Work out the finished part from the listing and answer in its coordinate system (mm). Round coordinates to 2 decimals unless told otherwise and drop trailing zeros. Write each loop counter-clockwise with the first axis right and the second up, starting at its lowest first coordinate (ties: lowest second). Pieces come first, ordered by that corner, then holes.
1. Find section B-B (y = -2). Write down the section's boundary in (x, z), and give its area (3 significant figures).
2. Find section C-C (z = 1.75). Count the separate pieces of the cut face and the enclosed holes in it, and give its area (3 significant figures).
3. Find section A-A (x = -27.5). Write down the section's boundary in (y, z).
4. Determine the mould class of faces 1 (the face through (-1, 23, 3)), 2 (the face through (-26.577, 29.726, 1.521)) for opening direction X: pulls with the +X half, pulls with the -X half, needs draft (parallel to the pull), parting line crosses it, or undercut.
5. Straight lines are drawn through the part: probe 1 along Y at (x, z) = (12, 1.15); probe 2 along X at (y, z) = (13, 2.75); probe 3 along Y at (x, z) = (-90, 1.2). For each, find the intervals that lie inside material, in ascending order.
Autodesk Inventor part; units mm, degrees
ref_plane "YZ Plane" through (0, 0, 0) normal (1, 0, 0) x (0, 1, 0)
ref_plane "XZ Plane" through (0, 0, 0) normal (0, 1, 0) x (-1, 0, 0)
ref_plane "XY Plane" through (0, 0, 0) normal (0, 0, 1) x (1, 0, 0)
sketch "Эскиз1" plane through (0, 0, 0) normal (0, 0, 1) x (1, 0, 0)
  line L0 (-100, -50) -> (100, -50)
  line L1 (100, -50) -> (100, 50)
  line L2 (100, 50) -> (-100, 50)
  line L3 (-100, 50) -> (-100, -50)
  line L4 (-100, -50) -> (100, 50) construction
  line L5 (100, -50) -> (-100, 50) construction
  line L6 (-45, -15) -> (45, -15) construction
  line L7 (45, -15) -> (45, 15) construction
  line L8 (45, 15) -> (-45, 15) construction
  line L9 (-45, 15) -> (-45, -15) construction
  line L10 (-45, -15) -> (45, 15) construction
  line L11 (45, -15) -> (-45, 15) construction
  line L12 (0, 15) -> (0, 18) construction
  line L13 (-45, 15) -> (-48, 15) construction
  line L14 (48, -18) -> (-48, -18)
  line L15 (-48, -18) -> (-48, 18)
  line L16 (-48, 18) -> (48, 18)
  line L17 (48, 18) -> (48, -18)
  line L18 (48, -18) -> (-48, 18) construction
  line L19 (-48, -18) -> (48, 18) construction
  point P0 (0, 0)
  dimension "d0" = 200
  dimension "d1" = 100
  dimension "d2" = 90
  dimension "d3" = 30
  dimension "d4" = 3
  dimension "d5" = 3
extrude "Выдавливание1" add sketch "Эскиз1" along normal blind 3
ref_plane "РабПлоскость1" through (0, -50, 0) normal (1, 0, 0) x (0, 0, -1)
sketch "Эскиз2" plane through (0, 0, 3) normal (0, 0, 1) x (1, 0, 0)
  line L0 (-48, -18) -> (-48, 18)
  line L1 (-48, 18) -> (48, 18)
  line L2 (48, 18) -> (48, -18)
  line L3 (48, -18) -> (-48, -18)
  line L4 (-100, -50) -> (100, -50)
  line L5 (100, -50) -> (100, 50)
  line L6 (100, 50) -> (-100, 50)
  line L7 (-100, 50) -> (-100, -50)
  line L8 (48, 18) -> (33.5, 18) construction
  line L9 (33.5, 18) -> (33.5, 50) construction
  line L10 (33.5, 18) -> (27.5, 18) construction
  line L11 (48, 18) -> (-48, 18) construction
  line L12 (27.5, 18) -> (27.5, 50) construction
  line L13 (100, 50) -> (-100, 50) construction
  line L14 (27.5, 18) -> (27.5, 24) construction
  circle A0 centre (27.5, 24) radius 2
  circle A1 centre (27.5, 31.5) radius 2
  circle A2 centre (27.5, 39) radius 2
  line L15 (0, 18) -> (0, 50)
  line L16 (-33.5, 18) -> (-27.5, 18) construction
  line L17 (-27.5, 18) -> (-27.5, 24) construction
  circle A3 centre (-27.5, 24) radius 2
  circle A4 centre (-27.5, 31.5) radius 2
  circle A5 centre (-27.5, 39) radius 2
  point P0 (0, 0)
  dimension "d8" = 14.5
  dimension "d9" = 6
  dimension "d10" = 6
  dimension "d11" = 4
  dimension "d14" = 7.5
extrude "Выдавливание2" cut sketch "Эскиз2" against normal blind 10 contours A0 | A1 | A2 | A3 | A4 | A5
sketch "Эскиз3" plane through (0, 0, 3) normal (0, 0, 1) x (1, 0, 0)
  circle A0 centre (-27.5, 31.5) radius 2
  circle A1 centre (27.5, 39) radius 2
  circle A2 centre (27.5, 24) radius 2
  circle A3 centre (27.5, 31.5) radius 2
  circle A4 centre (-27.5, 24) radius 2
  circle A5 centre (-27.5, 39) radius 2
  line L0 (-48, -18) -> (-48, 18)
  line L1 (-48, 18) -> (48, 18)
  line L2 (48, 18) -> (48, -18)
  line L3 (48, -18) -> (-48, -18)
  line L4 (-100, -50) -> (100, -50)
  line L5 (100, -50) -> (100, 50)
  line L6 (100, 50) -> (-100, 50)
  line L7 (-100, 50) -> (-100, -50)
  line L8 (-100, 50) -> (-90, 50) construction
  line L9 (-90, 50) -> (-90, 40) construction
  line L10 (-90, 40) -> (-100, 40) construction
  line L11 (-100, 40) -> (-100, 50) construction
  circle A6 centre (-90, 40) radius 1.5
  line L12 (-100, 50) -> (-100, -50)
  line L13 (-100, 0) -> (100, 0)
  line L14 (100, -50) -> (100, 50)
  line L15 (100, 50) -> (-100, 50)
  line L16 (0, 50) -> (0, -50)
  line L17 (-100, -50) -> (100, -50)
  circle A7 centre (90, 40) radius 1.5
  line L18 (0, -50) -> (0, -40) construction
  circle A8 centre (0, -40) radius 1.5
  point P0 (0, 0)
  dimension "d21" = 10
  dimension "d22" = 10
  dimension "d23" = 3
  dimension "d24" = 10
  dimension "d25" = 3
extrude "Выдавливание3" cut sketch "Эскиз3" against normal blind 10 contours A8 L16 | L16 A8 | A6 | A7
properties part number "Up Base"
Worked answers:
1. outline: (-100, 0) - (-48, 0) - (-48, 3) - (-100, 3) - close; (48, 0) - (100, 0) - (100, 3) - (48, 3) - close
1. area: 312 mm2
2. separate pieces: 1
2. enclosed holes: 10
2. area: 16,400 mm2
3. outline: (-50, 0) - (-18, 0) - (-18, 3) - (-50, 3) - close; (18, 0) - (22, 0) - (22, 3) - (18, 3) - close; (26, 0) - (29.5, 0) - (29.5, 3) - (26, 3) - close; (33.5, 0) - (37, 0) - (37, 3) - (33.5, 3) - close; (41, 0) - (50, 0) - (50, 3) - (41, 3) - close
4. face 1: needs draft
4. face 2: undercut
5. probe 1: y = -50 to -18, 18 to 50
5. probe 2: x = -100 to -48, 48 to 100
5. probe 3: y = -50 to 38.5, 41.5 to 50
